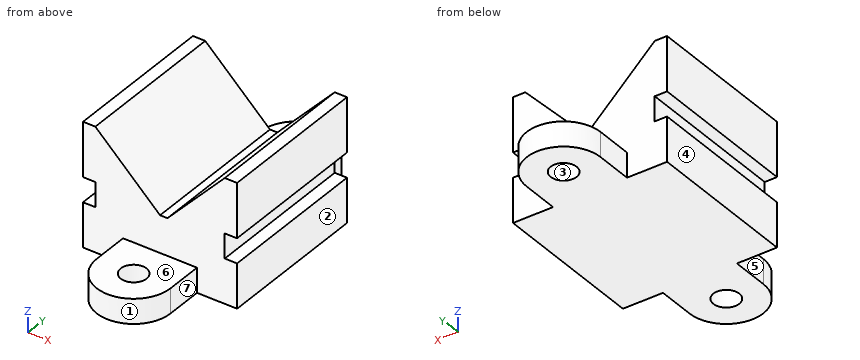
from build123d import *

# Parameters (mm, degrees)
F1_DEPTH = 62.5
F2_R     = 10.5
F3_DEPTH = 20


with BuildPart() as f1:
    # F0 (on Front) → F1 (new body, symmetric)
    with BuildSketch(Plane.XZ):
        Polygon((0, 0), (125, 0), (125, 36), (115, 36), (115, 56), (125, 56), (125, 100), (115, 100), (68.5, 50), (62.5, 50), (10, 100), (0, 100), (0, 56), (10, 56), (10, 36), (0, 36), align=None)
    extrude(amount=F1_DEPTH, both=True)

    # F2 (on Top) → F3 (join)
    with BuildSketch(Plane.XY):
        with BuildLine():
            Line((62.5, -62.5), (32.5, -62.5))
            Line((32.5, -62.5), (32.5, -92.5))
            ThreePointArc((32.5, -92.5), (62.5, -122.5), (92.5, -92.5))
            Line((92.5, -92.5), (92.5, -62.5))
            Line((92.5, -62.5), (62.5, -62.5))
        make_face()
        with Locations((62.5, -92.5)):
            Circle(F2_R, mode=Mode.SUBTRACT)
        with BuildLine():
            Line((32.5, 92.5), (32.5, 62.5))
            Line((32.5, 62.5), (62.5, 62.5))
            Line((62.5, 62.5), (92.5, 62.5))
            Line((92.5, 62.5), (92.5, 92.5))
            ThreePointArc((92.5, 92.5), (62.5, 122.5), (32.5, 92.5))
        make_face()
        with Locations((62.5, 92.5)):
            Circle(F2_R, mode=Mode.SUBTRACT)
    extrude(amount=F3_DEPTH)


solid = f1.part
Source: CAD feature listing. Evaluate the final solid. Frame: model axes, mm. Face numbers are marked on the shaded views. A direction names the side the tool comes from. Round coordinates to 2 decimals unless told otherwise and drop trailing zeros. Write each loop counter-clockwise with the first axis right and the second up, starting at its lowest first coordinate (ties: lowest second). Pieces come first, ordered by that corner, then holes. Notation, with made-up numbers: (65, 12) - (124, 12) arc R12 cw to (124, 32) - close; hole circle Ø10 at (89.5, 40). An arc over 180 degrees is marked (long way). Use CSV: the item, a comma, the result in double quotes. Start each with the question number.
(1) Set-up query: the marked faces 5, 6 and 7. Return all of +Z, -Z, +X, -X, +Y, -Y with unobstructed straight access to the full face (end or side cutting, diameter ignored); none if empty.
(2) Cut plane B-B, the plane z = 11. Return loops of the section in (x, y).
(3) Cut plane D-D, the plane y = 28. Return loops of the section in (x, z), and give its area (4 significant figures).
(4) Mould query, pull axis X, two halves, no side actions, for the marked faces 1, 2, 3 and 4. Classes: pulls with the +X half, pulls with the -X half, needs draft (parallel to the pull), parting line crosses it, or undercut.
(5) Material intervals for probe 1 along Y at (x, z) = (62, 12); probe 2 along X at (y, z) = (-92, 10); probe 3 along Y at (x, z) = (72, 17.5), sorted ascending. Write a range as [from, to].
(6) First-contact query: pin 1 Ø24 at (x, y) = (62.5, 92.5) entering from +Z; pin 2 Ø12 at (y, z) = (-15.5, 28) entering from -X; pin 3 Ø10 at (y, z) = (72, 5.5) entering from -X; pin 4 Ø1 at (x, z) = (95.5, 68.5) entering from -Y. Flat tips, straight axial feed; report the tip coordinate or a pass-through.
(7) Cut plane C-C, the plane y = 88. Return loops of the section in (x, z).
(8) Cut plane A-A, the plane z = 88. Return loops of the section in (x, y).
Geometry says:
1,face 5,"+Z, -Z, -X, -Y"
1,face 6,"+Z, +X, -X, -Y"
1,face 7,"+Z, -Z, +X, -Y"
2,outline,"(0, -62.5) - (32.5, -62.5) - (32.5, -92.5) arc R30 ccw to (92.5, -92.5) - (92.5, -62.5) - (125, -62.5) - (125, 62.5) - (92.5, 62.5) - (92.5, 92.5) arc R30 ccw to (32.5, 92.5) - (32.5, 62.5) - (0, 62.5) - close; hole circle Ø21 at (62.5, -92.5); hole circle Ø21 at (62.5, 92.5)"
3,outline,"(0, 0) - (125, 0) - (125, 36) - (115, 36) - (115, 56) - (125, 56) - (125, 100) - (115, 100) - (68.5, 50) - (62.5, 50) - (10, 100) - (0, 100) - (0, 56) - (10, 56) - (10, 36) - (0, 36) - close"
3,area,"9,325 mm²"
4,face 1,"parting line crosses it"
4,face 2,"pulls with the +X half"
4,face 3,"undercut"
4,face 4,"pulls with the -X half"
5,probe 1,"[-122.5, -102.99], [-82.01, 82.01], [102.99, 122.5]"
5,probe 2,"[32.5, 52.01], [72.99, 92.5]"
5,probe 3,"[-120.96, -96.97], [-88.03, 88.03], [96.97, 120.96]"
6,pin 1,"z = 20"
6,pin 2,"x = 0"
6,pin 3,"x = 32.5"
6,pin 4,"y = -62.5"
7,outline,"(32.5, 0) - (53.01, 0) - (53.01, 20) - (32.5, 20) - close; (71.99, 0) - (92.5, 0) - (92.5, 20) - (71.99, 20) - close"
8,outline,"(0, -62.5) - (22.6, -62.5) - (22.6, 62.5) - (0, 62.5) - close; (103.84, -62.5) - (125, -62.5) - (125, 62.5) - (103.84, 62.5) - close"
